```python
from build123d import *

# Parameters (mm, degrees)
ESQUISSE1_W                = 189
ESQUISSE1_H                = 73
BOSS_EXTRU_1_DEPTH         = 10
ESQUISSE2_W                = 10
ESQUISSE2_H                = 10
ENL_V_MAT_EXTRU_2_DEPTH    = 10
R_P_TITION_LIN_AIRE2_COUNT = 8
R_P_TITION_LIN_AIRE2_PITCH = 20
ESQUISSE3_W                = 30
ESQUISSE3_H                = 10
ENL_V_MAT_EXTRU_3_DEPTH    = 10
ESQUISSE4_W                = 10
ESQUISSE4_H                = 63
BOSS_EXTRU_2_DEPTH         = 83
ESQUISSE5_W                = 30
ESQUISSE5_H                = 10
BOSS_EXTRU_3_DEPTH         = 20
ESQUISSE6_R                = 5
ENL_V_MAT_EXTRU_4_DEPTH    = 10


with BuildPart() as part:
    # Esquisse1 → Boss.-Extru.1 (new body)
    with BuildSketch(Plane.XY):
        with Locations((-94.5, 36.5)):
            Rectangle(ESQUISSE1_W, ESQUISSE1_H)
    extrude(amount=BOSS_EXTRU_1_DEPTH)

    # Esquisse2 → Enlèv. mat.-Extru.2 (cut)
    with BuildSketch(Plane.XY.offset(10)):
        with Locations((-154, 5)):
            Rectangle(ESQUISSE2_W, ESQUISSE2_H)
    enl_v_mat_extru_2 = extrude(amount=-ENL_V_MAT_EXTRU_2_DEPTH, mode=Mode.SUBTRACT)

    # Répétition linéaire2: Enlèv. mat.-Extru.2 ×8
    with Locations(*[(i * R_P_TITION_LIN_AIRE2_PITCH, 0, 0) for i in range(1, R_P_TITION_LIN_AIRE2_COUNT)]):
        add(enl_v_mat_extru_2, mode=Mode.SUBTRACT)

    # Esquisse3 → Enlèv. mat.-Extru.3 (cut)
    with BuildSketch(Plane.XY.offset(10)):
        with Locations((-174, 5)):
            Rectangle(ESQUISSE3_W, ESQUISSE3_H)
    extrude(amount=-ENL_V_MAT_EXTRU_3_DEPTH, mode=Mode.SUBTRACT)

    # Esquisse4 → Boss.-Extru.2 (add)
    with BuildSketch(Plane(origin=(0, 0, 0), x_dir=(0, 0, -1), z_dir=(1, 0, 0))):
        with Locations((-5, 41.5)):
            Rectangle(ESQUISSE4_W, ESQUISSE4_H)
    extrude(amount=BOSS_EXTRU_2_DEPTH)

    # Esquisse5 → Boss.-Extru.3 (add)
    with BuildSketch(Plane.XZ.offset(-10)):
        with Locations((68, 5)):
            Rectangle(ESQUISSE5_W, ESQUISSE5_H)
    extrude(amount=BOSS_EXTRU_3_DEPTH)

    # Esquisse6 → Enlèv. mat.-Extru.4 (cut)
    with BuildSketch(Plane.XY.offset(10)):
        with Locations((68, 5)):
            Circle(ESQUISSE6_R)
    extrude(amount=-ENL_V_MAT_EXTRU_4_DEPTH, mode=Mode.SUBTRACT)


solid = part.part
```
Design review of the part built by this model. Coordinates are the model's own, in mm. A direction names the side the tool comes from. Round coordinates to 2 decimals unless told otherwise and drop trailing zeros. Order: outer loops, then holes, each group sorted by start corner. A loop starts at its lowest first (then second) coordinate and runs counter-clockwise, first axis right, second up. Notation, with made-up numbers: (10.25, 88) - (65.25, 88) arc R23 ccw to (65.25, 108) - close; hole circle Ø6 at (-26, -16.75). An arc over 180 degrees is marked (long way). Return JSON: item names as keys, results as strings.
Q1. For pin 1 Ø5 at (x, z) = (-124.5, 3.5) entering from -Y; pin 2 Ø5 at (y, z) = (6.5, 5.5) entering from -X; pin 3 Ø3 at (x, z) = (-56, 5) entering from -Y, all flat-tipped, find the tip position at first contact; note any pin that passes through.
Computed values:
{"pin 1": "stops at y = 0", "pin 2": "stops at x = -149", "pin 3": "stops at y = 10"}
Q2. The part is to be moulded in two halves that separate along X. For faces 1 (the flat face through (-74, 10, 5)), 2 (the flat face through (-104, 0, 5)), say which applies: pulls with the +X half, pulls with the -X half, needs draft (parallel to the pull), parting line crosses it, or undercut.
Computed values:
{"face 1": "undercut", "face 2": "needs draft"}
Q3. Machinability: for faces 3 (the flat face through (-94, 10, 5)), 4 (the flat face through (-64, 0, 5)), 5 (the flat face through (-55, 41, 10)), which of the approach directions +Z, -Z, +X, -X, +Y, -Y give a long, thin tool a straight path to every point of the face, cutting with its end or side? Answer none if there is none.
Computed values:
{"face 3": "+Z, -Z, -Y", "face 4": "+Z, -Z, -X, -Y", "face 5": "+Z, +X, -X, +Y, -Y"}
Q4. Consider section B-B on y = 5. Give the number of separate pieces and of enclosed holes in the cut face, plus the area to 3 significant figures.
Computed values:
{"separate pieces": "10", "enclosed holes": "0", "area": "990 mm2"}
Q5. Consider section A-A on x = 68. Write out the cut boundary in (y, z).
Computed values:
{"outline": "(-10, 0) - (0, 0) - (0, 10) - (-10, 10) - close; (10, 0) - (73, 0) - (73, 10) - (10, 10) - close"}
Q6. Consider section D-D on x = 13.5. Write out the cut boundary in (y, z).
Computed values:
{"outline": "(10, 0) - (73, 0) - (73, 10) - (10, 10) - close"}
Q7. Consider section C-C on x = -142.5. Write out the cut boundary in (y, z).
Computed values:
{"outline": "(0, 0) - (73, 0) - (73, 10) - (0, 10) - close"}
Q8. Wall thickness on L1, parallel to Y at x = 68, z = 7.75; L2, parallel to Y at x = -62, z = 8.25; L3, parallel to Y at x = -58, z = 8.5: over which ranges is each line inside the solid? List them lowest first. Write a range as [from, to].
Computed values:
{"L1": "y = [-10, 0], [10, 73]", "L2": "y = [0, 73]", "L3": "y = [10, 73]"}
